```python
from build123d import *

# Parameters (mm, degrees)
SKETCH1_W           = 76.2
SKETCH1_H           = 177.8
BOSS_EXTRUDE1_DEPTH = 4.7625
CUT_EXTRUDE1_REACH  = 98.838
SKETCH2_R           = 20.6375
CUT_EXTRUDE2_REACH  = 98.838
SKETCH4_R           = 3.175


with BuildPart() as part:
    # Sketch1 → Boss-Extrude1 (new body)
    with BuildSketch(Plane(origin=(0, 0, 0), x_dir=(0, 0, -1), z_dir=(1, 0, 0))):
        Rectangle(SKETCH1_W, SKETCH1_H)
    extrude(amount=BOSS_EXTRUDE1_DEPTH)

    # Sketch2 → Cut-Extrude1 (cut, up to next)
    with BuildSketch(Plane(origin=(4.7625, 0, 0), x_dir=(0, 0, -1), z_dir=(1, 0, 0)), mode=Mode.PRIVATE) as cut_extrude1_sk1:
        with Locations((0, 39.116)):
            Circle(SKETCH2_R)
    cut_extrude1_tool1 = extrude(cut_extrude1_sk1.sketch, amount=-CUT_EXTRUDE1_REACH, mode=Mode.PRIVATE) & part.part
    add(cut_extrude1_tool1.solids().sort_by_distance((4.7625, 39.116, 0))[0], mode=Mode.SUBTRACT)

    # Sketch4 → Cut-Extrude2 (cut, up to next)
    with BuildSketch(Plane(origin=(4.7625, 0, 0), x_dir=(0, 0, -1), z_dir=(1, 0, 0)), mode=Mode.PRIVATE) as cut_extrude2_sk1:
        with Locations((-19.05, -50.8)):
            Circle(SKETCH4_R)
    cut_extrude2_tool1 = extrude(cut_extrude2_sk1.sketch, amount=-CUT_EXTRUDE2_REACH, mode=Mode.PRIVATE) & part.part
    # Sketch4 → Cut-Extrude2 (cut, up to next)
    with BuildSketch(Plane(origin=(4.7625, 0, 0), x_dir=(0, 0, -1), z_dir=(1, 0, 0)), mode=Mode.PRIVATE) as cut_extrude2_sk2:
        with Locations((19.05, -50.8)):
            Circle(SKETCH4_R)
    cut_extrude2_tool2 = extrude(cut_extrude2_sk2.sketch, amount=-CUT_EXTRUDE2_REACH, mode=Mode.PRIVATE) & part.part
    # Sketch4 → Cut-Extrude2 (cut, up to next)
    with BuildSketch(Plane(origin=(4.7625, 0, 0), x_dir=(0, 0, -1), z_dir=(1, 0, 0)), mode=Mode.PRIVATE) as cut_extrude2_sk3:
        with Locations((19.05, -69.85)):
            Circle(SKETCH4_R)
    cut_extrude2_tool3 = extrude(cut_extrude2_sk3.sketch, amount=-CUT_EXTRUDE2_REACH, mode=Mode.PRIVATE) & part.part
    # Sketch4 → Cut-Extrude2 (cut, up to next)
    with BuildSketch(Plane(origin=(4.7625, 0, 0), x_dir=(0, 0, -1), z_dir=(1, 0, 0)), mode=Mode.PRIVATE) as cut_extrude2_sk4:
        with Locations((-19.05, -69.85)):
            Circle(SKETCH4_R)
    cut_extrude2_tool4 = extrude(cut_extrude2_sk4.sketch, amount=-CUT_EXTRUDE2_REACH, mode=Mode.PRIVATE) & part.part
    add(cut_extrude2_tool1.solids().sort_by_distance((4.7625, -50.8, 19.05))[0], mode=Mode.SUBTRACT)
    add(cut_extrude2_tool2.solids().sort_by_distance((4.7625, -50.8, -19.05))[0], mode=Mode.SUBTRACT)
    add(cut_extrude2_tool3.solids().sort_by_distance((4.7625, -69.85, -19.05))[0], mode=Mode.SUBTRACT)
    add(cut_extrude2_tool4.solids().sort_by_distance((4.7625, -69.85, 19.05))[0], mode=Mode.SUBTRACT)


solid = part.part
```
Read the model definition and answer for the solid it produces. Units are mm, in the model's axes. Give positions to 0.01 mm unless a question says otherwise; leave off trailing zeros. Write each loop counter-clockwise with the first axis right and the second up, starting at its lowest first coordinate (ties: lowest second). Pieces come first, ordered by that corner, then holes. Notation, with made-up numbers: (-6, 1) - (16, 1) arc R22 cw to (16, 9) - close; hole circle Ø11 at (60.25, 16.25). An arc over 180 degrees is marked (long way). Write item = value, one per line. Start each with the question number.
Item 1: The mould has two halves that part along Z. Classify faces 1 (the cylindrical face through (2.41, 18.97, 4.47)), 2 (the flat face through (2, -1, 38.1)), 3 (the flat face through (2, -88.9, 1)): +Z half, -Z half, draft (parallel to the pull), parting line (faces both ways), or undercut.
Item 2: Find section B-B (y = -50.8). Give the vertices of the cut face in (x, z) (1 decimal), then the cut area to 3 significant figures.
Item 3: Find section C-C (x = 1.4). State how many separate pieces and enclosed holes the cut face has, then the cut area to 3 significant figures.
Item 4: Find section A-A (z = 0). Give the vertices of the cut face in (x, y), then the cut area to 3 significant figures.
Item 5: Find section D-D (z = -19.05). Give the vertices of the cut face in (x, y) (1 decimal).
Item 6: Find the intervals of material crossed by probe 1 along Y at (x, z) = (1.6, 19.05) (1 decimal); probe 2 along Y at (x, z) = (1.15, 0); probe 3 along Y at (x, z) = (4.05, -1), in increasing order. Write a range as [from, to].
Response:
q1.face_1 = undercut
q1.face_2 = +Z half
q1.face_3 = draft
q2.outline = (0, -38.1) - (4.8, -38.1) - (4.8, -22.2) - (0, -22.2) - close; (0, -15.9) - (4.8, -15.9) - (4.8, 15.9) - (0, 15.9) - close; (0, 22.2) - (4.8, 22.2) - (4.8, 38.1) - (0, 38.1) - close
q2.area = 302 mm²
q3.separate_pieces = 1
q3.enclosed_holes = 5
q3.area = 12,100 mm²
q4.outline = (0, -88.9) - (4.76, -88.9) - (4.76, 18.48) - (0, 18.48) - close; (0, 59.75) - (4.76, 59.75) - (4.76, 88.9) - (0, 88.9) - close
q4.area = 650 mm²
q5.outline = (0, -88.9) - (4.8, -88.9) - (4.8, -73) - (0, -73) - close; (0, -66.7) - (4.8, -66.7) - (4.8, -54) - (0, -54) - close; (0, -47.6) - (4.8, -47.6) - (4.8, 31.2) - (0, 31.2) - close; (0, 47.1) - (4.8, 47.1) - (4.8, 88.9) - (0, 88.9) - close
q6.probe_1 = [-88.9, -73], [-66.7, -54], [-47.6, 31.2], [47.1, 88.9]
q6.probe_2 = [-88.9, 18.48], [59.75, 88.9]
q6.probe_3 = [-88.9, 18.5], [59.73, 88.9]
